from build123d import *

# Parameters (mm, degrees)
F0_R     = 1.5
F1_DEPTH = 1.5
F2_DEPTH = 8
F3_R     = 8
F4_R     = 3
F5_R     = 2
F6_R     = 8
F7_R     = 3
F8_R     = 2


with BuildPart() as f1:
    # F0 (on Front) → F1 (new body)
    with BuildSketch(Plane.XZ):
        with BuildLine():
            Line((-26.0642077774, -18.5), (-18.8888516277, -18.5))
            Line((-18.8888516277, -18.5), (-18.8888516277, -14))
            ThreePointArc((-18.8888516277, -14), (-23.3701047123, 0), (-18.8888516277, 14))
            Line((-18.8888516277, 14), (-18.8888516277, 18.5))
            Line((-18.8888516277, 18.5), (-25.6080199033, 18.5))
            Line((-25.6080199033, 18.5), (-37.3901407018, 5.4135240382))
            ThreePointArc((-37.3901407018, 5.4135240382), (-28.5949290555, 7.4538958141), (-23.5, 0))
            ThreePointArc((-23.5, 0), (-28.6715728753, -7.4833147735), (-37.5, -5.2915026221))
            Line((-37.5, -5.2915026221), (-37.5, -5.2920114501))
            Line((-37.5, -5.2920114501), (-26.0642077774, -18.5))
        make_face()
        with Locations((-22.5, -15.25)):
            Circle(F0_R, mode=Mode.SUBTRACT)
        with Locations((-22.5, 15.25)):
            Circle(F0_R, mode=Mode.SUBTRACT)
    extrude(amount=F1_DEPTH)

    # F0 (on Front) → F2 (join)
    with BuildSketch(Plane.XZ):
        with BuildLine():
            Line((-37.5, 0), (-37.5, -5.2915026221))
            ThreePointArc((-37.5, -5.2915026221), (-28.6715728753, -7.4833147735), (-23.5, 0))
            ThreePointArc((-23.5, 0), (-28.5949290555, 7.4538958141), (-37.3901407018, 5.4135240382))
            Line((-37.3901407018, 5.4135240382), (-37.5, 5.2915026221))
            Line((-37.5, 5.2915026221), (-37.5, 0))
        make_face()
        with BuildLine():
            ThreePointArc((-25.5, 0), (-31.5, -6), (-37.5, 0))
            ThreePointArc((-37.5, 0), (-31.5, 6), (-25.5, 0))
        make_face(mode=Mode.SUBTRACT)
        with BuildLine():
            ThreePointArc((-37.5, 5.2915026221), (-39.5, 0), (-37.5, -5.2915026221))
            Line((-37.5, -5.2915026221), (-37.5, 0))
            Line((-37.5, 0), (-37.5, 5.2915026221))
        make_face()
    extrude(amount=F2_DEPTH)

    # F3
    f3_edges = [f1.edges().sort_by_distance(p)[0] for p in [
        (-26.064208, -0.75, -18.5),
    ]]
    fillet(f3_edges, radius=F3_R)

    # F4
    f4_edges = [f1.edges().sort_by_distance(p)[0] for p in [
        (-18.888852, -0.75, -18.5),
    ]]
    fillet(f4_edges, radius=F4_R)

    # F5
    f5_edges = [f1.edges().sort_by_distance(p)[0] for p in [
        (-18.888852, -0.75, 14),
    ]]
    fillet(f5_edges, radius=F5_R)

    # F6
    f6_edges = [f1.edges().sort_by_distance(p)[0] for p in [
        (-25.60802, -0.75, 18.5),
    ]]
    fillet(f6_edges, radius=F6_R)

    # F7
    f7_edges = [f1.edges().sort_by_distance(p)[0] for p in [
        (-18.888852, -0.75, 18.5),
    ]]
    fillet(f7_edges, radius=F7_R)

    # F8
    f8_edges = [f1.edges().sort_by_distance(p)[0] for p in [
        (-18.888852, -0.75, -14),
    ]]
    fillet(f8_edges, radius=F8_R)


solid = f1.part
Geometry: final body of the model. Coordinates: model frame, mm. A direction names the side the tool comes from. Coordinates: 2 decimals unless noted, no trailing zeros. Write each loop counter-clockwise with the first axis right and the second up, starting at its lowest first coordinate (ties: lowest second). Pieces come first, ordered by that corner, then holes. Notation, with made-up numbers: (-23.5, 72.25) - (23.5, 72.25) arc R24 cw to (23.5, 91.25) - close; hole circle Ø4 at (52.5, 71). An arc over 180 degrees is marked (long way). Return JSON: item names as keys, results as strings.
Item 1: Pin query (flat end, axial travel): pin 1 Ø4 at (x, z) = (-22.5, 15.25) entering from -Y; pin 2 Ø1.5 at (x, y) = (-33.5, -3) entering from -Z; pin 3 Ø4 at (x, z) = (-22.5, -15.25) entering from +Y. Return the tip coordinate at first contact, or that it passes through.
Completed:
{"pin 1": "stops at y = -1.5", "pin 2": "stops at z = -7.9", "pin 3": "stops at y = 0"}
Item 2: Section query B-B (y = -1). Count the separate pieces of the cut face and the enclosed holes in it, and give its area (3 significant figures).
Completed:
{"separate pieces": "1", "enclosed holes": "3", "area": "329 mm2"}
Item 3: Reachability of faces 4 (the face through (-18.98, -0.76, 14.03)), 5 (the face through (-25.257, -0.76, 17.827)) from +Z, -Z, +X, -X, +Y, -Y: full face, straight path, thin tool, end or side. Return the list, or none.
Completed:
{"face 4": "+X, +Y, -Y", "face 5": "+Z, -X, +Y, -Y"}
Item 4: Section query D-D (x = -34.25). Output: boundary loops of the cut face in (y, z).
Completed:
{"outline": "(-8, -7.51) - (-1.5, -7.51) - (-1.5, -9.05) - (0, -9.05) - (0, -5.33) - (-8, -5.33) - close; (-8, 5.33) - (0, 5.33) - (0, 8.9) - (-1.5, 8.9) - (-1.5, 7.51) - (-8, 7.51) - close"}
Item 5: Section query C-C (y = -4). Output: boundary loops of the cut face in (x, z), and give its area (3 significant figures).
Completed:
{"outline": "(-37.5, 5.29) arc R8 ccw (long way) to (-37.39, 5.41) - close; hole circle Ø12 at (-31.5, 0)", "area": "88.0 mm2"}
Item 6: Line query: L1, parallel to Z at x = -31.5, y = -3.5; L2, parallel to Z at x = -30.5, y = -0.25; L3, parallel to Y at x = -31.25, z = -11.5. Output: solid intervals per line, ascending.
Completed:
{"L1": "z = -8 to -6, 6 to 8", "L2": "z = -13.38 to -5.92, 5.92 to 13.07", "L3": "y = -1.5 to 0"}
Item 7: Pull-direction query (Z, two-part tool) for faces 1 (the face through (-24, -0.7, -15.2)), 2 (the face through (-25, 0, 0)), 3 (the face through (-19.791, -0.76, -17.645)); classes: +Z half, -Z half, draft (parallel to the pull), parting line (faces both ways), or undercut.
Completed:
{"face 1": "undercut", "face 2": "draft", "face 3": "-Z half"}
Item 8: Section query A-A (x = -31). Output: boundary loops of the cut face in (y, z).
Completed:
{"outline": "(-8, -7.98) - (-1.5, -7.98) - (-1.5, -12.8) - (0, -12.8) - (0, -5.98) - (-8, -5.98) - close; (-8, 5.98) - (0, 5.98) - (0, 12.51) - (-1.5, 12.51) - (-1.5, 7.98) - (-8, 7.98) - close"}
